Build history of the part. All positions in model axes, mm. A direction names the side the tool comes from. Give positions to 0.01 mm unless a question says otherwise; leave off trailing zeros. Loops run counter-clockwise (first coordinate to the right, second up) from the corner with the lowest first, then second, coordinate; pieces in that order, holes last. Notation, with made-up numbers: (-18.75, -10) -> (31.25, -10) arc R32 ccw to (31.25, 17) -> close; hole circle Ø8 at (86.5, 83). An arc over 180 degrees is marked (long way). One line per question, with ' | ' between items. Start each with the question number.
(1) Mould opens along X. For faces 3 (the face through (12.7, -125, 0)), 4 (the face through (0, -129, -11.112)), 5 (the face through (-11.348, -4.726, 0.059)) say: pulls with the +X half, pulls with the -X half, needs draft (parallel to the pull), parting line crosses it, or undercut.
(2) Slice it at A-A, the plane x = -7.5. Write the cut outline in (y, z).
(3) Flat gauge pin, fed straight in: pin 1 Ø12 at (x, z) = (6, 8.5) entering from -Y. Where does the tip first touch, or does it go through?
(4) Drill centre lines: L1, parallel to X at y = -58.5, z = 4; L2, parallel to Y at x = 11.75, z = -5.25. Where is each one in solid material? Low to high. Write a range as from..to.
(5) 3-axis set-ups, long thin cutter, end or side, ignore diameter. For faces 1 (the face through (0, -121, 12.7)), 2 (the face through (11.112, -125, 0)): which of +Z, -Z, +X, -X, +Y, -Y reach the whole face in a straight line?
(6) Slice it at C-C, the plane z = -3.75. Write the cut outline in (x, y).
(7) Slice it at B-B, the plane y = -211.5. Write the cut outline in (x, z), then the cut area to 3 significant figures.
```python
from build123d import *

# Parameters (mm, degrees)
F0_W        = 25.4
F0_H        = 25.4
F0_W_2      = 22.225
F0_H_2      = 22.225
F1_DEPTH    = 254
F2_T1_DEPTH = 157.170304922
F3_T1_DEPTH = 157.170304922


# Not quite as in the source:
# - a fillet or chamfer that OpenCascade refuses, or shapes differently, is made with other operations: its cross-section is extruded or revolved along the edge and cut away or added


with BuildPart() as f1:
    # F0 (on Front) → F1 (new body)
    with BuildSketch(Plane.XZ):
        Rectangle(F0_W, F0_H)
        Rectangle(F0_W_2, F0_H_2, mode=Mode.SUBTRACT)
    extrude(amount=F1_DEPTH)

    # F2: chamfer of 25.4 x 9.4966708589 on 1 edges, made by hand

    # F2_s2 → F2_t1 (cut)
    with BuildSketch(Plane.YZ.offset(-78.585152461)):
        Polygon((-244.5033291411, 12.7), (-254, -12.7), (-254, 12.7), align=None)
    extrude(amount=F2_T1_DEPTH, mode=Mode.SUBTRACT)

    # F3: chamfer of 25.4 x 9.4966708589 on 1 edges, made by hand

    # F3_s2 → F3_t1 (cut)
    with BuildSketch(Plane.YZ.offset(-78.585152461)):
        Polygon((0, 12.7), (-9.4966708589, -12.7), (0, -12.7), align=None)
    extrude(amount=F3_T1_DEPTH, mode=Mode.SUBTRACT)


solid = f1.part
```
Final values:
1) face 3: pulls with the +X half | face 4: undercut | face 5: needs draft
2) outline: (-254, -12.7) -> (-9.5, -12.7) -> (-8.9, -11.11) -> (-253.41, -11.11) -> close; (-245.1, 11.11) -> (-0.59, 11.11) -> (0, 12.7) -> (-244.5, 12.7) -> close
3) pin 1: y = -247.25
4) L1: -12.7..-11.11, 11.11..12.7 | L2: -251.21..-6.71
5) face 1: +Z, +X, -X, +Y, -Y | face 2: +Y, -Y
6) outline: (-12.7, -250.65) -> (-11.11, -250.65) -> (-11.11, -6.15) -> (-12.7, -6.15) -> close; (11.11, -250.65) -> (12.7, -250.65) -> (12.7, -6.15) -> (11.11, -6.15) -> close
7) outline: (-12.7, -12.7) -> (12.7, -12.7) -> (12.7, 12.7) -> (-12.7, 12.7) -> close; hole (-11.11, -11.11) -> (11.11, -11.11) -> (11.11, 11.11) -> (-11.11, 11.11) -> close | area: 151 mm2
